Could you check a few things on this model? Use its own coordinates, in mm. A direction names the side the tool comes from. Round coordinates to 2 decimals unless told otherwise and drop trailing zeros. Write each loop counter-clockwise with the first axis right and the second up, starting at its lowest first coordinate (ties: lowest second). Pieces come first, ordered by that corner, then holes. Notation, with made-up numbers: (30, 5) -> (35, 5) arc R16 cw to (35, 11) -> close; hole circle Ø7 at (9.5, 34.25). An arc over 180 degrees is marked (long way). Return JSON: item names as keys, results as strings.
Autodesk Inventor part; units mm, degrees
ref_plane "作業平面1" through (0, 0, 12) normal (0, 0, 1) x (1, 0, 0)
ref_plane "YZ Plane" through (0, 0, 0) normal (1, 0, 0) x (0, 1, 0)
ref_plane "XZ Plane" through (0, 0, 0) normal (0, 1, 0) x (-1, 0, 0)
sketch "スケッチ1" plane through (0, 0, 0) normal (0, 0, 1) x (1, 0, 0)
  circle A0 centre (0, 0) radius 3
  circle A1 centre (0, 0) radius 1.5
  dimension "d0" = 6
  dimension "d1" = 3
extrude "押し出し1" add sketch "スケッチ1" along normal blind 18
ref_plane "作業平面1" through (0, 0, 12) normal (0, 0, 1) x (1, 0, 0)
sketch "スケッチ3" plane through (0, 0, 12) normal (0, 0, 1) x (1, 0, 0)
  circle A0 centre (0, 0) radius 1.5
  circle A1 centre (0, 0) radius 3
extrude "押し出し2" add sketch "スケッチ3" against normal blind 6 contours A0
properties part number "スペーサーm3-18　簡易筒型" material "アルミニウム 2014-T4"
1) I want a section at C-C, the plane z = 1.75. Please give me the cut outline in (x, y).
Return value:
{"outline": "circle Ø6 at (0, 0); hole circle Ø3 at (0, 0)"}
2) I want a section at D-D, the plane z = 11.25. Please give me the cut outline in (x, y).
Return value:
{"outline": "circle Ø6 at (0, 0)"}
3) Will these pins go through, and if not, where does the flat tip stop? pin 1 Ø1 at (x, z) = (-1, 13) entering from +Y; pin 2 Ø2.5 at (x, y) = (0, 0) entering from -Z; pin 3 Ø2.5 at (x, y) = (0, 0) entering from +Z.
Return value:
{"pin 1": "y = 2.96", "pin 2": "z = 6", "pin 3": "z = 12"}
4) For faces 4 (the face through (-1.5, -0.07, 2.96)), 5 (the face through (1.3, -1.3, 18)), 6 (the face through (-1.5, -0.07, 14.96)), which set-ups out of +Z, -Z, +X, -X, +Y, -Y let a thin tool reach every point of the face, with its end or its side?
Return value:
{"face 4": "-Z", "face 5": "+Z, +X, -X, +Y, -Y", "face 6": "+Z"}
5) I want a section at A-A, the plane y = 0. Please give me the cut outline in (x, z), and give its area (3 significant figures).
Return value:
{"outline": "(-3, 0) -> (-1.5, 0) -> (-1.5, 6) -> (1.5, 6) -> (1.5, 0) -> (3, 0) -> (3, 18) -> (1.5, 18) -> (1.5, 12) -> (-1.5, 12) -> (-1.5, 18) -> (-3, 18) -> close", "area": "72.0 mm²"}
6) If I drill on probe 1 along X at (y, z) = (-0.1, 15.5); probe 2 along Y at (x, z) = (0.9, 12.75), over which ranges is the centre line in solid material (lowest first)? Write a range as [from, to].
Return value:
{"probe 1": "[-3, -1.5], [1.5, 3]", "probe 2": "[-2.86, -1.2], [1.2, 2.86]"}
7) Thinking about a two-plate mould opening in Y: for faces 1 (the face through (0, 0, 12)), 2 (the face through (1.3, -1.3, 0)), 3 (the face through (-3, 0, 9)), which applies, pulls with the +Y half, pulls with the -Y half, needs draft (parallel to the pull), parting line crosses it, or undercut?
Return value:
{"face 1": "undercut", "face 2": "needs draft", "face 3": "parting line crosses it"}
